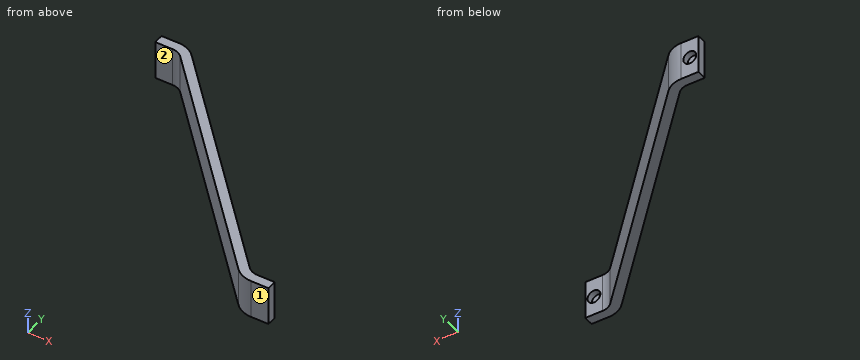
from build123d import *

# Parameters (mm, degrees)
SKETCH_2_W          = 60
SKETCH_2_H          = 15
SKETCH_3_R          = 10
CUT_EXTRUDE_1_DEPTH = 10
SKETCH_4_R          = 10
CUT_EXTRUDE_2_DEPTH = 10


with BuildPart() as part:
    # 扫描1: sweep along a path in 草图1
    with BuildLine(Plane.XY) as sweep_1_path:
        Line((0, 0), (26.862133413, 0))
        ThreePointArc((26.862133413, 0), (38.896590134, -2.519609693), (48.909571267, -9.655209904))
        Line((48.909571267, -9.655209904), (351.090428733, -337.125468596))
        ThreePointArc((351.090428733, -337.125468596), (361.103409866, -344.261068807), (373.137866587, -346.7806785))
        Line((373.137866587, -346.7806785), (400, -346.7806785))
    # 草图2 → 扫描1 (sweep)
    with BuildSketch(Plane(origin=(0, 0, 0), x_dir=(0, 0, -1), z_dir=(1, 0, 0))):
        Rectangle(SKETCH_2_W, SKETCH_2_H)
    sweep(path=sweep_1_path.line)

    # 草图3 → 切除-拉伸1 (cut)
    with BuildSketch(Plane(origin=(0, 7.5, 0), x_dir=(1, 0, 0), z_dir=(0, 1, 0))):
        with Locations(Location((13.431066706, 0, 0), (0, 0, 270))):
            Circle(SKETCH_3_R)
    extrude(amount=-CUT_EXTRUDE_1_DEPTH, mode=Mode.SUBTRACT)

    # 草图4 → 切除-拉伸2 (cut)
    with BuildSketch(Plane(origin=(0, -339.2806785, 0), x_dir=(1, 0, 0), z_dir=(0, 1, 0))):
        with Locations(Location((386.568933294, 0, 0), (0, 0, 180))):
            Circle(SKETCH_4_R)
    extrude(amount=-CUT_EXTRUDE_2_DEPTH, mode=Mode.SUBTRACT)


solid = part.part
The model under review builds one solid part; all positions refer to its coordinate system, in mm. Face numbers are marked on the shaded views. A direction names the side the tool comes from. Give positions to 0.01 mm unless a question says otherwise; leave off trailing zeros. Order: outer loops, then holes, each group sorted by start corner. A loop starts at its lowest first (then second) coordinate and runs counter-clockwise, first axis right, second up. Notation, with made-up numbers: M 50,-12 L 80,-12 A37 ccw 80,25 Z; hole C -10,13 d1. An arc over 180 degrees is marked long. Answer in a Markdown table with one row per item. Add a question column.
1. Add section C-C on x = 33.5. State the section outline as (y, z) points.
2. Add section A-A on z = 24. State the section outline as (x, y) points, plus the area to 3 significant figures.
3. For pin 1 Ø5 at (y, z) = (-231.5, 11.5) entering from -X; pin 2 Ø8 at (x, z) = (157.5, -15) entering from -Y; pin 3 Ø10 at (x, z) = (359, 0) entering from +Y; pin 4 Ø16 at (x, z) = (18, 2) entering from +Y, all flat-tipped, find the tip position at first contact; note any pin that passes through.
4. Add section D-D on y = -300. State the section outline as (x, z) points.
5. Machinability: for the marked faces 1 and 2, which of the approach directions +Z, -Z, +X, -X, +Y, -Y give a long, thin tool a straight path to every point of the face, cutting with its end or side? Answer none if there is none.
6. Add section B-B on z = 0. State the section outline as (x, y) points, plus the area to 3 significant figures.
7. To check wall thickness, follow line 1 along Y through (x, z) = (25, -1); line 2 along X through (y, z) = (1, 0); line 3 along Y through (x, z) = (382.5, 27). State the ranges of each line that lie inside material, in increasing order.
The answers:
| question | item | result |
|---|---|---|
| 1 | outline | M -8.5,-30 L 6.91,-30 L 6.91,30 L -8.5,30 Z |
| 2 | outline | M 0,-7.5 L 26.86,-7.5 A22.5 cw 43.4,-14.74 L 345.58,-342.21 A37.5 ccw 373.14,-354.28 L 400,-354.28 L 400,-339.28 L 373.14,-339.28 A22.5 cw 356.6,-332.04 L 54.42,-4.57 A37.5 ccw 26.86,7.5 L 0,7.5 Z |
| 2 | area | 8,230 mm2 |
| 3 | pin 1 | x = 241.11 |
| 3 | pin 2 | y = -142.73 |
| 3 | pin 3 | y = -329.22 |
| 3 | pin 4 | y = 7.5 |
| 4 | outline | M 306.63,-30 L 327.04,-30 L 327.04,30 L 306.63,30 Z |
| 5 | face 1 | +Z, -Z, +X, -X, -Y |
| 5 | face 2 | +Z, -Z, -X, -Y |
| 6 | outline | M 0,-7.5 L 26.86,-7.5 A22.5 cw 43.4,-14.74 L 345.58,-342.21 A37.5 ccw 373.14,-354.28 L 400,-354.28 L 400,-339.28 L 396.57,-339.28 L 396.57,-349.28 L 376.57,-349.28 L 376.57,-339.28 L 373.14,-339.28 A22.5 cw 356.6,-332.04 L 54.42,-4.57 A37.5 ccw 26.86,7.5 L 23.43,7.5 L 23.43,-2.5 L 3.43,-2.5 L 3.43,7.5 L 0,7.5 Z |
| 6 | area | 7,830 mm2 |
| 7 | line 1 | -7.5 to 7.5 |
| 7 | line 2 | 0 to 3.43, 23.43 to 47.96 |
| 7 | line 3 | -354.28 to -339.28 |
